```python
from build123d import *

# Parameters (mm, degrees)
SKETCH_W        = 40
SKETCH_H        = 47.5
PAD_DEPTH       = 12
SKETCH001_R     = 1.6
POCKET_DEPTH    = 8
SKETCH002_R     = 1.6
POCKET001_DEPTH = 8
SKETCH003_W     = 5.8
SKETCH003_H     = 3
POCKET002_DEPTH = 12
SKETCH004_R     = 1.6
POCKET003_DEPTH = 12
POCKET004_DEPTH = 9
POCKET005_DEPTH = 12
POCKET006_DEPTH = 50
FILLET_R        = 0.2


with BuildPart() as part:
    # Sketch → Pad (new body)
    with BuildSketch(Plane.XY):
        Rectangle(SKETCH_W, SKETCH_H)
    extrude(amount=PAD_DEPTH)

    # Sketch001 (on Face3 of Pad) → Pocket (cut)
    with BuildSketch(Plane.XZ.offset(23.75)):
        with Locations((-15, 6)):
            Circle(SKETCH001_R)
        with Locations((15, 6)):
            Circle(SKETCH001_R)
    extrude(amount=-POCKET_DEPTH, mode=Mode.SUBTRACT)

    # Sketch002 (on Face1 of Pocket) → Pocket001 (cut)
    with BuildSketch(Plane(origin=(0, 23.75, 0), x_dir=(-1, 0, 0), z_dir=(0, 1, 0))):
        with Locations((-15, 6)):
            Circle(SKETCH002_R)
        with Locations((15, 6)):
            Circle(SKETCH002_R)
    extrude(amount=-POCKET001_DEPTH, mode=Mode.SUBTRACT)

    # Sketch003 (on Face4 of Pocket001) → Pocket002 (cut)
    with BuildSketch(Plane.XY.offset(9.5)):
        with Locations((-15, 19.25)):
            Rectangle(SKETCH003_W, SKETCH003_H)
        with Locations((15, 19.25)):
            Rectangle(SKETCH003_W, SKETCH003_H)
        with Locations((-15, -19.25)):
            Rectangle(SKETCH003_W, SKETCH003_H)
        with Locations((15, -19.25)):
            Rectangle(SKETCH003_W, SKETCH003_H)
    extrude(amount=-POCKET002_DEPTH, mode=Mode.SUBTRACT)

    # Sketch004 (on Face4 of Pocket002) → Pocket003 (cut)
    with BuildSketch(Plane.XY.offset(12)):
        with Locations((-15, 5)):
            Circle(SKETCH004_R)
        with Locations((15, 5)):
            Circle(SKETCH004_R)
        with Locations((-15, -5)):
            Circle(SKETCH004_R)
        with Locations((15, -5)):
            Circle(SKETCH004_R)
    extrude(amount=-POCKET003_DEPTH, mode=Mode.SUBTRACT)

    # Sketch005 (on Face4 of Pocket003) → Pocket004 (cut)
    with BuildSketch(Plane.XY.offset(12)):
        Polygon((-15, 8.290897), (-17.85, 6.645448), (-17.85, 3.354552), (-15, 1.709103), (-12.15, 3.354552), (-12.15, 6.645448), align=None)
        Polygon((15, 8.290897), (12.15, 6.645448), (12.15, 3.354552), (15, 1.709103), (17.85, 3.354552), (17.85, 6.645448), align=None)
        Polygon((-15, -1.709103), (-17.85, -3.354552), (-17.85, -6.645448), (-15, -8.290897), (-12.15, -6.645448), (-12.15, -3.354552), align=None)
        Polygon((15, -1.709103), (12.15, -3.354552), (12.15, -6.645448), (15, -8.290897), (17.85, -6.645448), (17.85, -3.354552), align=None)
    extrude(amount=-POCKET004_DEPTH, mode=Mode.SUBTRACT)

    # Sketch006 → Pocket005 (cut)
    with BuildSketch(Plane.XY.offset(12)):
        with BuildLine():
            Line((-2.5, 12.5), (2.5, 12.5))
            ThreePointArc((7.5, 7.5), (6.035534, 11.035534), (2.5, 12.5))
            Line((7.5, 7.5), (7.5, -7.5))
            ThreePointArc((2.5, -12.5), (6.035534, -11.035534), (7.5, -7.5))
            Line((2.5, -12.5), (-2.5, -12.5))
            ThreePointArc((-7.5, -7.5), (-6.035534, -11.035534), (-2.5, -12.5))
            Line((-7.5, -7.5), (-7.5, 7.5))
            ThreePointArc((-2.5, 12.5), (-6.035534, 11.035534), (-7.5, 7.5))
        make_face()
    extrude(amount=-POCKET005_DEPTH, mode=Mode.SUBTRACT)

    # Sketch009 (on Face8 of Pocket005) → Pocket006 (cut)
    with BuildSketch(Plane.XZ.offset(23.75)):
        with BuildLine():
            ThreePointArc((-13, 12), (-17.949747, 9.949747), (-20, 5))
            Line((-20, 5), (-20, 13))
            Line((-20, 13), (20, 13))
            Line((20, 13), (20, 5))
            ThreePointArc((20, 5), (17.949747, 9.949747), (13, 12))
            Line((13, 12), (-13, 12))
        make_face()
    extrude(amount=-POCKET006_DEPTH, mode=Mode.SUBTRACT)

    # Fillet
    fillet_edges = [part.edges().sort_by_distance(p)[0] for p in [
        (20, -23.75, 2.5),
        (-20, -23.75, 2.5),
        (20, 23.75, 2.5),
        (-20, 23.75, 2.5),
    ]]
    fillet(fillet_edges, radius=FILLET_R)


solid = part.part
```
Work out the finished part from the listing and answer in its coordinate system (mm). A direction names the side the tool comes from. Coordinates: 2 decimals unless noted, no trailing zeros. Write each loop counter-clockwise with the first axis right and the second up, starting at its lowest first coordinate (ties: lowest second). Pieces come first, ordered by that corner, then holes. Notation, with made-up numbers: (-33, 84) - (-1, 84) arc R29 cw to (-1, 115) - close; hole circle Ø6 at (-17, 15.5). An arc over 180 degrees is marked (long way). Answer as a JSON object with one key per item and string values.
Q1. Which of the six approach directions +Z, -Z, +X, -X, +Y, -Y give full straight-line access (tool end or side, diameter ignored) to faces 4 (the flat face through (-15, -17.75, 4)), 5 (the flat face through (-15, -15.75, 6)), 6 (the flat face through (-16.44, -7.46, 7.42))?
Results list:
{"face 4": "-Z", "face 5": "-Y", "face 6": "+Z"}
Q2. For a pull along Y with two mould halves and no side action, classify faces 1 (the cylindrical face through (16.6, 22.27, 6.07)), 2 (the flat face through (0, -23.75, 6)), 3 (the flat face through (15, -17.75, 4)) as pulls with the +Y half, pulls with the -Y half, needs draft (parallel to the pull), parting line crosses it, or undercut.
Results list:
{"face 1": "needs draft", "face 2": "pulls with the -Y half", "face 3": "undercut"}
Q3. Find section B-B (y = 5). Write down the section's boundary in (x, z).
Results list:
{"outline": "(-20, 0) - (-16.6, 0) - (-16.6, 3) - (-17.85, 3) - (-17.85, 10.05) arc R7 ccw to (-20, 5) - close; (-13.4, 0) - (-7.5, 0) - (-7.5, 12) - (-12.15, 12) - (-12.15, 3) - (-13.4, 3) - close; (7.5, 0) - (13.4, 0) - (13.4, 3) - (12.15, 3) - (12.15, 12) - (7.5, 12) - close; (16.6, 0) - (20, 0) - (20, 5) arc R7 ccw to (17.85, 10.05) - (17.85, 3) - (16.6, 3) - close"}
Q4. Given pin 1 Ø2.5 at (x, y) = (-15.5, -20) entering from -Z; pin 2 Ø0.9 at (y, z) = (-19.5, 7) entering from -X; pin 3 Ø1.6 at (y, z) = (4.5, 9) entering from +X; pin 4 Ø1 at (x, z) = (-15.5, 5.5) entering from +Y, each flat-ended and moving along its own axis, determine where each tip first touches the part or whether it passes through.
Results list:
{"pin 1": "stops at z = 0", "pin 2": "stops at x = -19.83", "pin 3": "stops at x = 19.23", "pin 4": "stops at y = 15.75"}
Q5. Find section C-C (y = -19). Write down the section's boundary in (x, z).
Results list:
{"outline": "(-20, 0) - (-17.9, 0) - (-17.9, 9.5) - (-12.1, 9.5) - (-12.1, 0) - (12.1, 0) - (12.1, 9.5) - (17.9, 9.5) - (17.9, 0) - (20, 0) - (20, 5) arc R7 ccw to (13, 12) - (-13, 12) arc R7 ccw to (-20, 5) - close"}
Q6. Consider L1, parallel to Y at x = -15, z = 8.5; L2, parallel to Y at x = -15, z = 0.85; L3, parallel to Y at x = 2, z = 7. Determine where each line is inside the solid, lowest interval first. Write a range as from..to.
Results list:
{"L1": "y = -23.75..-20.75, -17.75..-8.29, -1.71..1.71, 8.29..17.75, 20.75..23.75", "L2": "y = -23.75..-20.75, -17.75..-6.6, -3.4..3.4, 6.6..17.75, 20.75..23.75", "L3": "y = -23.75..-12.5, 12.5..23.75"}
Q7. Find section D-D (x = 0.5). Write down the section's boundary in (y, z).
Results list:
{"outline": "(-23.75, 0) - (-12.5, 0) - (-12.5, 12) - (-23.55, 12) arc R0.2 ccw to (-23.75, 11.8) - close; (12.5, 0) - (23.75, 0) - (23.75, 11.8) arc R0.2 ccw to (23.55, 12) - (12.5, 12) - close"}
Q8. Find section A-A (x = -5.5). Write down the section's boundary in (y, z), plus the area to 3 significant figures.
Results list:
{"outline": "(-23.75, 0) - (-11.5, 0) - (-11.5, 12) - (-23.55, 12) arc R0.2 ccw to (-23.75, 11.8) - close; (11.5, 0) - (23.75, 0) - (23.75, 11.8) arc R0.2 ccw to (23.55, 12) - (11.5, 12) - close", "area": "294 mm^2"}
